from build123d import *

# Parameters (mm, degrees)
BOSS_EXTRUDE1_DEPTH = 30
CUT_EXTRUDE1_START  = -35
SKETCH2_R           = 2
CUT_EXTRUDE1_DEPTH  = 3
CUT_EXTRUDE2_START  = -3
SKETCH3_R           = 2
CUT_EXTRUDE2_DEPTH  = 3


with BuildPart() as part:
    # Sketch1 → Boss-Extrude1 (new body)
    with BuildSketch(Plane(origin=(0, 0, 0), x_dir=(1, 0, 0), z_dir=(0, 1, 0))):
        Polygon((0, 0), (-10, 0), (-10, 20), (25, 20), (25, 0), (15, 0), (15, 10), (20, 10), (20, 15), (-5, 15), (-5, 10), (0, 10), align=None)
    extrude(amount=BOSS_EXTRUDE1_DEPTH)

    # Sketch2 → Cut-Extrude1 (cut)
    with BuildSketch(Plane.ZY.offset(10).offset(CUT_EXTRUDE1_START)):
        with Locations((-13, 25)):
            Circle(SKETCH2_R)
        with Locations((-13, 5)):
            Circle(SKETCH2_R)
    extrude(amount=CUT_EXTRUDE1_DEPTH, mode=Mode.SUBTRACT)

    # Sketch3 → Cut-Extrude2 (cut)
    with BuildSketch(Plane.ZY.offset(10).offset(CUT_EXTRUDE2_START)):
        with Locations((-13, 25)):
            Circle(SKETCH3_R)
        with Locations((-13, 5)):
            Circle(SKETCH3_R)
    extrude(amount=CUT_EXTRUDE2_DEPTH, mode=Mode.SUBTRACT)


solid = part.part
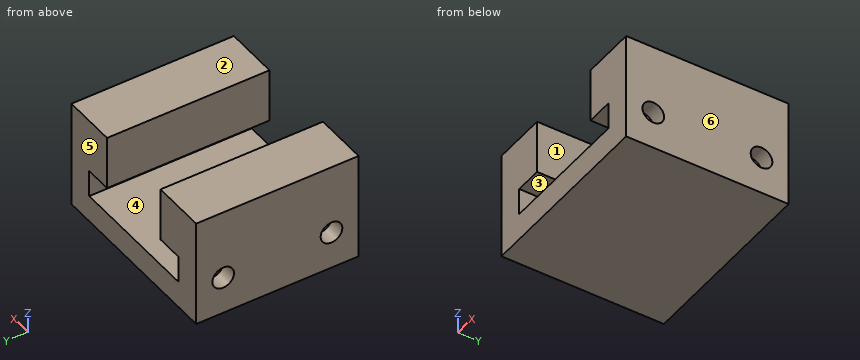
Geometry: final body of the model. Coordinates: model frame, mm. Face numbers are marked on the shaded views. A direction names the side the tool comes from. Give positions to 0.01 mm unless a question says otherwise; leave off trailing zeros. Write each loop counter-clockwise with the first axis right and the second up, starting at its lowest first coordinate (ties: lowest second). Pieces come first, ordered by that corner, then holes. Notation, with made-up numbers: (-3.75, -40) -> (52.25, -40) arc R33 ccw to (52.25, -3) -> close; hole circle Ø3 at (28, 14). An arc over 180 degrees is marked (long way). Answer in a Markdown table with one row per item.
(1) Section query B-B on x = -2. Return loops of the section in (y, z).
Answers below:
| item | result |
|---|---|
| outline | (0, -20) -> (30, -20) -> (30, -15) -> (0, -15) -> close; (0, -10) -> (30, -10) -> (30, 0) -> (0, 0) -> close |
(2) Pin query (flat end, axial travel): pin 1 (1.2 mm diameter, centred on y = 25, z = -13.5, fed in from -X); pin 2 (3 mm diameter, centred on y = 5, z = -13, fed in from +X); pin 3 (2 mm diameter, centred on y = 4, z = -13.5, fed in from +X). Return the tip coordinate at first contact, or that it passes through.
Answers below:
| item | result |
|---|---|
| pin 1 | x = -7 |
| pin 2 | x = 22 |
| pin 3 | x = 25 |
(3) Section query D-D on z = -13. Return loops of the section in (x, y), then the cut area to 3 significant figures.
Answers below:
| item | result |
|---|---|
| outline | (-10, 0) -> (-5, 0) -> (-5, 30) -> (-10, 30) -> (-10, 27) -> (-7, 27) -> (-7, 23) -> (-10, 23) -> (-10, 7) -> (-7, 7) -> (-7, 3) -> (-10, 3) -> close; (20, 0) -> (25, 0) -> (25, 3) -> (22, 3) -> (22, 7) -> (25, 7) -> (25, 23) -> (22, 23) -> (22, 27) -> (25, 27) -> (25, 30) -> (20, 30) -> close |
| area | 252 mm^2 |
(4) Set-up query: the marked faces 1, 2 and 3. Return all of +Z, -Z, +X, -X, +Y, -Y with unobstructed straight access to the full face (end or side cutting, diameter ignored); none if empty.
Answers below:
| item | result |
|---|---|
| face 1 | +Z, +Y, -Y |
| face 2 | +Z, +X, -X, +Y, -Y |
| face 3 | +Y, -Y |
(5) Section query A-A on z = -7. Return loops of the section in (x, y).
Answers below:
| item | result |
|---|---|
| outline | (-10, 0) -> (0, 0) -> (0, 30) -> (-10, 30) -> close; (15, 0) -> (25, 0) -> (25, 30) -> (15, 30) -> close |
(6) Draft query along X for the marked faces 4, 5 and 6. Return one class per face: +X half, -X half, draft (parallel to the pull), parting line (faces both ways), or undercut.
Answers below:
| item | result |
|---|---|
| face 4 | undercut |
| face 5 | draft |
| face 6 | +X half |
(7) Ray query, line 1 along Y through (x, z) = (-8.5, -13); line 2 along X through (y, z) = (10.5, -10.25); line 3 along Z through (x, y) = (-0.5, 28). Return the intervals inside material, ascending. Write a range as [from, to].
Answers below:
| item | result |
|---|---|
| line 1 | [0, 3], [7, 23], [27, 30] |
| line 2 | [-10, -5], [20, 25] |
| line 3 | [-20, -15], [-10, 0] |
(8) Section query C-C on y = 25. Return loops of the section in (x, z).
Answers below:
| item | result |
|---|---|
| outline | (-10, -20) -> (25, -20) -> (25, -15) -> (22, -15) -> (22, -11) -> (25, -11) -> (25, 0) -> (15, 0) -> (15, -10) -> (20, -10) -> (20, -15) -> (-5, -15) -> (-5, -10) -> (0, -10) -> (0, 0) -> (-10, 0) -> (-10, -11) -> (-7, -11) -> (-7, -15) -> (-10, -15) -> close |
